```python
from build123d import *

# Parameters (mm, degrees)
F1_DEPTH = 38.1
F2_R     = 31.878636
F3_DEPTH = 127
F4_SIZE  = 5.08
F5_R     = 21.263534
F6_DEPTH = 127


with BuildPart() as f1:
    # F0 (on Front) → F1 (new body)
    with BuildSketch(Plane.XZ):
        Polygon((39.800733, -52.655495), (65.501363, 8.140698), (25.70063, 60.796193), (-39.800733, 52.655495), (-65.501363, -8.140698), (-25.70063, -60.796193), align=None)
    extrude(amount=F1_DEPTH)

    # F2 (on face) → F3 (join)
    with BuildSketch(Plane.XZ.offset(38.1)):
        Circle(F2_R)
    extrude(amount=F3_DEPTH)

    # F4
    f4_edges = [f1.edges().sort_by_distance(p)[0] for p in [
        (-31.878636, -165.1, 0),
    ]]
    chamfer(f4_edges, length=F4_SIZE)

    # F5 (on face) → F6 (join)
    with BuildSketch(Plane.XZ.offset(165.1)):
        Circle(F5_R)
    extrude(amount=F6_DEPTH)


solid = f1.part
```
The listing builds one solid part. Answer for the finished solid, in the listing's coordinates (mm). A direction names the side the tool comes from. Give positions to 0.01 mm unless a question says otherwise; leave off trailing zeros. Loops run counter-clockwise (first coordinate to the right, second up) from the corner with the lowest first, then second, coordinate; pieces in that order, holes last. Notation, with made-up numbers: (61.5, -1.5) - (77.5, -1.5) arc R32 ccw to (77.5, 28.5) - close; hole circle Ø3 at (-27, 56.5). An arc over 180 degrees is marked (long way). Return JSON: item names as keys, results as strings. Group by question number.
1. Find section A-A (z = 0). Write down the section's boundary in (x, y), then the cut area to 3 significant figures.
2. Find section D-D (y = -20.5). Write down the section's boundary in (x, z), then the cut area to 3 significant figures.
3. Straight lines are drawn through the part: line 1 (Y direction, x = 48, z = 18); line 2 (X direction, y = -227, z = 10); line 3 (X direction, y = -34, z = -23.5). For each, find the intervals that lie inside material, in ascending order. Write a range as [from, to].
4. Which of the six approach directions +Z, -Z, +X, -X, +Y, -Y give full straight-line access (tool end or side, diameter ignored) to faces 1 (the flat face through (-52.471, -18.783, 22.683)), 2 (the cylindrical face through (17.14, -98.21, 26.88))?
5. Find section C-C (y = -129.5). Write down the section's boundary in (x, z).
6. Given pin 1 Ø12 at (x, y) = (25.5, -207) entering from -Z; pin 2 Ø6 at (x, y) = (-7.5, -78) entering from +Z; pin 3 Ø1 at (x, z) = (-24.5, -47) entering from -Y, each flat-ended and moving along its own axis, determine where each tip first touches the part or whether it passes through.
7. Find section B-B (x = 0). Write down the section's boundary in (y, z), then the cut area to 3 significant figures.
Verdict:
{
 "1": {"outline": "(-62.06, -38.1) - (-31.88, -38.1) - (-31.88, -160.02) - (-26.8, -165.1) - (-21.26, -165.1) - (-21.26, -292.1) - (21.26, -292.1) - (21.26, -165.1) - (26.8, -165.1) - (31.88, -160.02) - (31.88, -38.1) - (62.06, -38.1) - (62.06, 0) - (-62.06, 0) - close", "area": "18,200 mm^2"},
 "2": {"outline": "(-65.5, -8.14) - (-25.7, -60.8) - (39.8, -52.66) - (65.5, 8.14) - (25.7, 60.8) - (-39.8, 52.66) - close", "area": "11,300 mm^2"},
 "3": {"line 1": "y = [-38.1, 0]", "line 2": "x = [-18.77, 18.77]", "line 3": "x = [-53.89, 52.13]"},
 "4": {"face 1": "+Z, -X, +Y, -Y", "face 2": "-Y"},
 "5": {"outline": "circle Ø63.76 at (0, 0)"},
 "6": {"pin 1": "stops at z = -8.48", "pin 2": "stops at z = 31.56", "pin 3": "stops at y = -38.1"},
 "7": {"outline": "(-292.1, -21.26) - (-165.1, -21.26) - (-165.1, -26.8) - (-160.02, -31.88) - (-38.1, -31.88) - (-38.1, -57.6) - (0, -57.6) - (0, 57.6) - (-38.1, 57.6) - (-38.1, 31.88) - (-160.02, 31.88) - (-165.1, 26.8) - (-165.1, 21.26) - (-292.1, 21.26) - close", "area": "17,900 mm^2"}
}
